For this review, take the finished solid that the model builds, in its own axes (mm). Face numbers are marked on the shaded views. A direction names the side the tool comes from. Coordinates: 2 decimals unless noted, no trailing zeros. Write each loop counter-clockwise with the first axis right and the second up, starting at its lowest first coordinate (ties: lowest second). Pieces come first, ordered by that corner, then holes. Notation, with made-up numbers: (77, 13.5) - (110, 13.5) arc R16 cw to (110, 43.5) - close; hole circle Ø9 at (78, 2). An arc over 180 degrees is marked (long way). Use one line per item in the form item = value. Start each with the question number.
1) Mouldability with a two-part tool opening along Z and no side actions: class the marked faces 4, 5 and 6 as pulls with the +Z half, pulls with the -Z half, needs draft (parallel to the pull), parting line crosses it, or undercut.
2) Tool access review of the marked faces 1, 2 and 3: name each direction out of +Z, -Z, +X, -X, +Y, -Y from which nothing blocks a thin tool from reaching the whole face with its end or side.
3) Insertion check: P1, Ø13, axis at x = 17.5, y = 50, coming from the -Z side; P2, Ø21, axis at x = 127.5, y = 21.5, coming from the +Z side; P3, Ø2, axis at x = 47.5, y = 60, coming from the +Z side; P4, Ø15, axis at x = 58, y = 38.5, coming from the -Z side. Each pin has a flat end and moves straight along its axis. Give the tip position at first contact, or say it passes through.
4) For L1, parallel to Z at x = 52, y = 23.5; L2, parallel to X at y = 45, z = 54.5; L3, parallel to Z at x = 23, y = 40.5, list the stretches that pass through material, from the lowest coordinate up. Write a range as from..to.
5) We need section C-C (y = 30). Give the boundary of the cut face in (x, z).
6) We need section A-A (z = 67). Give the boundary of the cut face in (x, y).
7) We need section B-B (x = 81). Give the boundary of the cut face in (y, z), plus the area to 3 significant figures.
8) We need section D-D (y = 58.5). Give the boundary of the cut face in (x, z), plus the area to 3 significant figures.
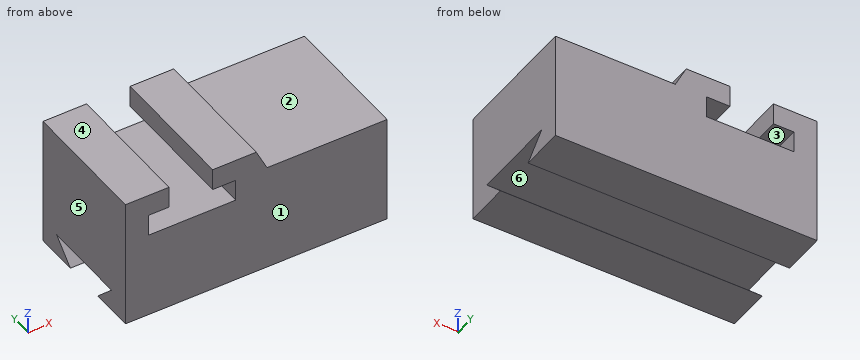
```python
from build123d import *

# Parameters (mm, degrees)
F0_W      = 152.4
F0_H      = 76.2
F1_DEPTH  = 76.2
F3_DEPTH  = 152.4
F4_W      = 69.85
F4_H      = 12.7
F5_DEPTH  = 76.2
F7_DEPTH  = 76.2
F8_W      = 25.4
F8_H      = 12.7
F9_DEPTH  = 76.2
F11_DEPTH = 76.2


# Not quite as in the source:
# - a feature names something its author has since deleted; it is built from what else it names


with BuildPart() as f1:
    # F0 (on Front) → F1 (new body)
    with BuildSketch(Plane.XZ):
        with Locations((76.2, 38.1)):
            Rectangle(F0_W, F0_H)
    extrude(amount=-F1_DEPTH)

    # F2 (on face) → F3 (cut)
    with BuildSketch(Plane.YZ.offset(152.4)):
        Polygon((25.5270022899, 0), (38.1, 0), (50.9269982576, 0), (63.6270046234, 12.573000975), (12.8270015121, 12.573000975), align=None)
    extrude(amount=-F3_DEPTH, mode=Mode.SUBTRACT)

    # F4 (on face) → F5 (cut)
    with BuildSketch(Plane.XZ):
        with Locations((117.475, 69.85)):
            Rectangle(F4_W, F4_H)
    extrude(amount=-F5_DEPTH, mode=Mode.SUBTRACT)

    # F6 (on face) → F7 (cut)
    with BuildSketch(Plane.XZ):
        Polygon((76.2, 76.2), (82.55, 63.5), (82.55, 76.2), align=None)
    extrude(amount=-F7_DEPTH, mode=Mode.SUBTRACT)

    # F8 (on face) → F9 (cut)
    with BuildSketch(Plane.XZ):
        with Locations((38.1, 69.85)):
            Rectangle(F8_W, F8_H)
    extrude(amount=-F9_DEPTH, mode=Mode.SUBTRACT)

    # F10 (on face) → F11 (cut)
    with BuildSketch(Plane.XZ):
        Polygon((64.2725850075, 63.5), (38.1, 63.5), (13.4725850075, 63.5), (13.4725850075, 50.8), (64.2725850075, 50.8), align=None)
    extrude(amount=-F11_DEPTH, mode=Mode.SUBTRACT)


solid = f1.part
```
Determined:
q1.face_4 = pulls with the +Z half
q1.face_5 = needs draft
q1.face_6 = undercut
q2.face_1 = +Z, -Z, +X, -X, -Y
q2.face_2 = +Z, +X, +Y, -Y
q2.face_3 = +Y, -Y
q3.P1 = 0
q3.P2 = 63.5
q3.P3 = 50.8
q3.P4 = 12.57
q4.L1 = 0..2.01, 12.57..50.8, 63.5..76.2
q4.L2 = 0..13.47, 64.27..152.4
q4.L3 = 12.57..50.8, 63.5..76.2
q5.outline = (0, 12.57) - (152.4, 12.57) - (152.4, 63.5) - (82.55, 63.5) - (76.2, 76.2) - (50.8, 76.2) - (50.8, 63.5) - (64.27, 63.5) - (64.27, 50.8) - (13.47, 50.8) - (13.47, 63.5) - (25.4, 63.5) - (25.4, 76.2) - (0, 76.2) - close
q6.outline = (0, 0) - (25.4, 0) - (25.4, 76.2) - (0, 76.2) - close; (50.8, 0) - (80.8, 0) - (80.8, 76.2) - (50.8, 76.2) - close
q7.outline = (0, 0) - (25.53, 0) - (12.83, 12.57) - (63.63, 12.57) - (50.93, 0) - (76.2, 0) - (76.2, 66.6) - (0, 66.6) - close
q7.area = 4,600 mm²
q8.outline = (0, 0) - (152.4, 0) - (152.4, 7.5) - (0, 7.5) - close; (0, 12.57) - (152.4, 12.57) - (152.4, 63.5) - (82.55, 63.5) - (76.2, 76.2) - (50.8, 76.2) - (50.8, 63.5) - (64.27, 63.5) - (64.27, 50.8) - (13.47, 50.8) - (13.47, 63.5) - (25.4, 63.5) - (25.4, 76.2) - (0, 76.2) - close
q8.area = 8,940 mm²
